Autodesk Fusion 360 part; units mm, degrees
sketch "Sketch1" plane through (0, 0, 0) normal (0, 0, 1) x (1, 0, 0)
  line L0 (-21.8, 22.2397) -> (26.7, 22.2397)
  line L1 (26.7, 22.2397) -> (26.7, -22.7603)
  line L2 (26.7, -22.7603) -> (-21.8, -22.7603)
  line L3 (-21.8, -22.7603) -> (-21.8, 22.2397)
  spline S0 degree 5 poles (-8.2949, 12.4487) (-8.8839, 11.9576) (-10.0102, 10.9741) (-11.5448, 9.495) (-13.2761, 7.5148) (-14.8799, 5.0253) (-15.8741, 2.5205) (-16.2099, -0.001) (-15.8626, -2.5398) (-14.8614, -5.0951) (-13.2565, -7.6657) (-11.5298, -9.7334) (-10.0015, -11.2901) (-8.8808, -12.3304) (-8.2949, -12.8513) knots 0 0 0 0 0 0 0.1 0.2 0.3 0.4 0.5 0.6 0.7 0.8 0.9 1 1 1 1 1 1
  spline S1 degree 5 poles (14.2993, 7.4153) (14.5562, 7.1034) (15.0477, 6.4806) (15.718, 5.5494) (16.4756, 4.3142) (17.1805, 2.7814) (17.6209, 1.2609) (17.7748, -0.2462) (17.6287, -1.7394) (17.193, -3.2192) (16.4888, -4.6864) (15.7281, -5.8511) (15.0535, -6.7197) (14.5583, -7.2967) (14.2993, -7.5847) knots 0 0 0 0 0 0 0.1 0.2 0.3 0.4 0.5 0.6 0.7 0.8 0.9 1 1 1 1 1 1
  line L4 (-21.8, -1.6206) -> (-14.6097, -1.6206)
  line L5 (-14.6097, -1.6206) -> (-14.6097, 0.3794)
  line L6 (-14.6097, 0.3794) -> (-21.8, 0.3794)
  line L7 (14.2993, 7.4153) -> (0.6904, 13.733)
  line L8 (0.6904, 13.733) -> (-8.2949, 12.4487)
  line L9 (0.4715, -12.8513) -> (-8.2949, -12.8513)
  line L10 (14.2993, -7.5847) -> (8.5702, -10.0161)
  line L11 (8.5702, -10.0161) -> (0.4715, -12.8513)
  point P0 (-16.0393, 0.095)
  point P1 (17.6997, -0.3339)
  dimension "d6" = 48.5
  dimension "d7" = 45
  dimension "d8" = 15
  dimension "d9" = 25.3
  dimension "d11" = 2
extrude "Extrude1" add sketch "Sketch1" along normal blind 35.3 contours L0 L1 L2 L3 S0 S1 L4 L6 L7 L8 L9 L10 L11
sketch "bad_sketch" plane through (0, 0, 0) normal (0, 0, 1) x (1, 0, 0)
  line L0 (24.6924, 6.1679) -> (15.4617, 8.9936)
  line L1 (15.4617, 8.9936) -> (5.166, 12.1454)
  line L2 (5.166, 12.1454) -> (-5.166, 12.8182)
  line L3 (-5.166, 12.8182) -> (-14.9618, 9.182)
  line L4 (-14.9618, 9.182) -> (-20.3307, 2.1177)
  line L5 (-20.3307, 2.1177) -> (-20.3307, -2.686)
  line L6 (-20.3307, -2.686) -> (-14.9618, -8.9968)
  line L7 (-14.9618, -8.9968) -> (-10.0639, -11.3515)
  line L8 (-10.0639, -11.3515) -> (-5.166, -12.4818)
  line L9 (-5.166, -12.4818) -> (5.166, -12.4818)
  line L10 (5.166, -12.4818) -> (10.3139, -11.0689)
  line L11 (10.3139, -11.0689) -> (24.6924, -8.2432)
  line L12 (24.6924, -8.2432) -> (28.2717, -1.8383)
  line L13 (28.2717, -1.8383) -> (28.9264, 0.3007)
  line L14 (28.9264, 0.3007) -> (26.482, 5.6201)
  line L15 (26.482, 5.6201) -> (24.6924, 6.1679)
  line L16 (-28.837, -17.65) -> (19.663, -17.65)
  line L17 (19.663, -17.65) -> (19.663, 27.35)
  line L18 (19.663, 27.35) -> (-28.837, 27.35)
  line L19 (-28.837, 27.35) -> (-28.837, -17.65)
  line L20 (-28.837, -1.4888) -> (-19.0112, -1.4888)
  line L21 (-19.0112, -1.4888) -> (-19.0112, 0.5112)
  line L22 (-19.0112, 0.5112) -> (-28.837, 0.5112)
  line L23 (-28.837, 0.5112) -> (-28.837, -1.4888)
  dimension "d15" = 48.5
  dimension "d16" = 45
  dimension "d17" = 2
sketch "Sketch3" plane through (0, 22.2397, 0) normal (0, 1, 0) x (-1, 0, 0)
  line L0 (-26.7, 0) -> (21.8, 0)
  line L1 (21.8, 0) -> (21.8, 35.3)
  line L2 (21.8, 35.3) -> (-26.7, 35.3)
  line L3 (-26.7, 35.3) -> (-26.7, 0)
  circle A0 centre (18.6487, 11.1813) radius 1.7
  line L4 (21.8, 13.5098) -> (16.4, 13.5098)
  line L5 (16.4, 13.5098) -> (16.4, 8.2098)
  line L6 (16.4, 8.2098) -> (21.8, 8.2098)
  line L7 (21.8, 8.2098) -> (21.8, 13.5098)
  dimension "d23" = 3.4
  dimension "d26" = 5.4
  dimension "d27" = 5.3
hole "Hole1" at (-18.6487, 22.2397, 11.1813) direction (0, -1, 0) diameter 3.4 depth 26 tip angle 180
extrude "Extrude3" cut sketch "Sketch3" against normal blind 16 contours L1 L4 L5 L6 L7
sketch "Sketch4" plane through (0, -22.7603, 0) normal (0, -1, 0) x (1, 0, 0)
  line L0 (-21.8, 0) -> (26.7, 0)
  line L1 (26.7, 0) -> (26.7, 35.3)
  line L2 (26.7, 35.3) -> (-21.8, 35.3)
  line L3 (-21.8, 35.3) -> (-21.8, 0)
  line L4 (18.0274, 30.3462) -> (-12.9426, 30.3462)
  line L5 (18.0274, 30.3462) -> (18.0274, 5.3462)
  line L6 (18.0274, 5.3462) -> (-12.9426, 5.3462)
  circle A0 centre (18.0274, 5.3462) radius 1.6
  circle A1 centre (-12.9426, 5.3462) radius 1.6
  circle A2 centre (18.0274, 30.3462) radius 1.6
  circle A3 centre (-12.9426, 30.3462) radius 1.6
  line L7 (26.7, 14.5722) -> (17.935, 14.5722)
  dimension "d36" = 30.97
  dimension "d38" = 25
  dimension "d40" = 30.97
  dimension "d41" = 3.2
  dimension "d42" = 3.2
  dimension "d43" = 3.2
  dimension "d44" = 3.2
  dimension "d45" = 8.765
hole "Hole2" at (18.0274, -22.7603, 5.3462) at (-12.9426, -22.7603, 5.3462) at (18.0274, -22.7603, 30.3462) at (-12.9426, -22.7603, 30.3462) direction (0, 1, 0) diameter 3.2 depth 12 tip angle 180
sketch "Sketch5" plane through (-21.8, 0, 0) normal (-1, 0, 0) x (0, -1, 0)
  line L0 (1.6206, 0) -> (22.7603, 0)
  line L1 (22.7603, 0) -> (22.7603, 35.3)
  line L2 (22.7603, 35.3) -> (1.6206, 35.3)
  line L3 (1.6206, 35.3) -> (1.6206, 0)
  line L4 (22.7603, 16.2062) -> (19.7603, 16.2062)
  line L5 (19.7603, 7.0647) -> (16.0603, 7.0647)
  line L6 (16.0603, 7.0647) -> (16.0603, 1.8647)
  line L7 (16.0603, 1.8647) -> (19.7603, 1.8647)
  line L8 (19.7603, 1.8647) -> (19.7603, 7.0647)
  line L9 (19.7603, 27.5787) -> (16.0603, 27.5787)
  line L10 (16.0603, 27.5787) -> (16.0603, 32.7787)
  line L11 (16.0603, 32.7787) -> (19.7603, 32.7787)
  line L12 (19.7603, 32.7787) -> (19.7603, 27.5787)
  line L13 (6.4749, 8.7948) -> (2.7749, 8.7948)
  line L14 (2.7749, 8.7948) -> (2.7749, 13.9948)
  line L15 (2.7749, 13.9948) -> (6.4749, 13.9948)
  line L16 (6.4749, 13.9948) -> (6.4749, 8.7948)
  dimension "d55" = 3
  dimension "d56" = 3.7
  dimension "d57" = 5.2
  dimension "d58" = 3.7
  dimension "d59" = 5.2
  dimension "d65" = 3.7
  dimension "d66" = 5.2
extrude "Extrude4" cut sketch "Sketch5" against normal blind 12 contours L9 L10 L11 L12
extrude "Extrude5" cut sketch "Sketch5" against normal blind 12 contours L5 L6 L7 L8
extrude "Extrude6" cut sketch "Sketch5" against normal blind 5.4 contours L13 L14 L15 L16
sketch "Sketch7" plane through (26.7, 0, 0) normal (1, 0, 0) x (0, 1, 0)
  line L0 (-22.7603, 0) -> (22.2397, 0)
  line L1 (22.2397, 0) -> (22.2397, 35.3)
  line L2 (22.2397, 35.3) -> (-22.7603, 35.3)
  line L3 (-22.7603, 35.3) -> (-22.7603, 0)
  line L4 (-19.7634, 32.4808) -> (-16.0634, 32.4808)
  line L5 (-16.0634, 32.4808) -> (-16.0634, 27.2808)
  line L6 (-16.0634, 27.2808) -> (-19.7634, 27.2808)
  line L7 (-19.7634, 27.2808) -> (-19.7634, 32.4808)
  line L8 (-19.7359, 7.0548) -> (-16.0359, 7.0548)
  line L9 (-16.0359, 7.0548) -> (-16.0359, 1.8548)
  line L10 (-16.0359, 1.8548) -> (-19.7359, 1.8548)
  line L11 (-19.7359, 1.8548) -> (-19.7359, 7.0548)
  dimension "d76" = 3.7
  dimension "d77" = 5.2
  dimension "d78" = 3.7
  dimension "d79" = 5.2
extrude "Extrude8" cut sketch "Sketch7" against normal blind 12 contours L4 L5 L6 L7 | L8 L9 L10 L11
equation "syringe_height = 25.3 mm"
equation "syringe_width = 33.6 mm"
equation "height = 45 mm"
equation "width = 48.5 mm"
equation "width4 = 15 mm"
equation "d6 = width"
equation "d7 = height"
equation "d8 = width4"
equation "d9 = syringe_height"
equation "gap_width = 2 mm"
equation "d11 = gap_width"
equation "d12 = holder_depth"
equation "d15 = width"
equation "d16 = height"
equation "d17 = gap_width"
equation "length = 3 mm"
equation "holder_depth = 35.3 mm"
equation "m3_screw_diameter = 3.4 mm"
equation "d23 = m3_screw_diameter"
equation "rect_clearing_width = 5.3 mm"
equation "rect_clearing_length = 5.4 mm"
equation "d26 = rect_clearing_length"
equation "d27 = rect_clearing_width"
equation "d28 = joining_m3_screw_length"
equation "d29 = m3_screw_diameter"
equation "joining_m3_screw_length = 26 mm"
equation "rect_clearing_distance = 16 mm"
equation "m3_screw_lateral_dis = 30.97 mm"
equation "d36 = m3_screw_lateral_dis"
equation "m3_screw_vertical_dis = 25 mm"
equation "d38 = m3_screw_vertical_dis"
equation "m3_diameter = 3.2 mm"
equation "d40 = m3_screw_lateral_dis"
equation "d41 = m3_diameter"
equation "d42 = m3_diameter"
equation "d43 = m3_diameter"
equation "d44 = m3_diameter"
equation "d46 = m3_screw_depth"
equation "d47 = m3_diameter"
equation "m3_screw_depth = 12 mm"
equation "nut_insert_width = 3.7 mm"
equation "nut_insert_height = 5.2 mm"
equation "screw_nut_distance = 3 mm"
equation "d55 = screw_nut_distance"
equation "d56 = nut_insert_width"
equation "d57 = nut_insert_height"
equation "d58 = nut_insert_width"
equation "d59 = nut_insert_height"
equation "d60 = -m3_screw_depth"
equation "d62 = -m3_screw_depth"
equation "d65 = nut_insert_width"
equation "d66 = nut_insert_height"
equation "clamp_nut_depth = 5.4 mm"
equation "d76 = nut_insert_width"
equation "d77 = nut_insert_height"
equation "d78 = nut_insert_width"
equation "d79 = nut_insert_height"
equation "d80 = -m3_screw_depth"
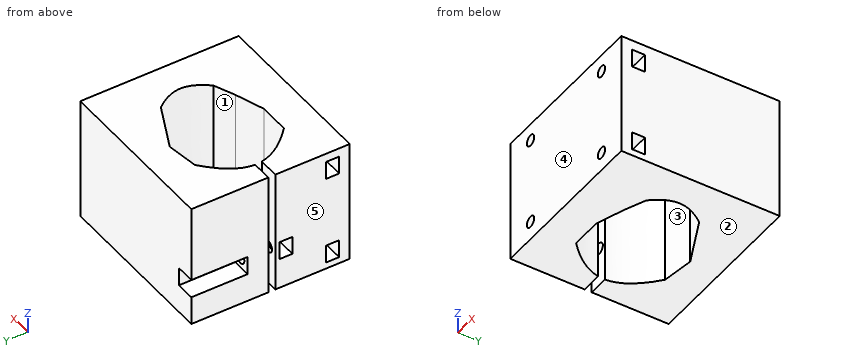
Verification items for the finished model (mm, model axes). Face numbers are marked on the shaded views. A direction names the side the tool comes from. Coordinates: 2 decimals unless noted, no trailing zeros. Order: outer loops, then holes, each group sorted by start corner. A loop starts at its lowest first (then second) coordinate and runs counter-clockwise, first axis right, second up. Notation, with made-up numbers: M 5.25,-21 L 64.25,-21 A19 ccw 64.25,6 Z; hole C 88.5,-9 d10. An arc over 180 degrees is marked long. One line per item, written item: value. Start each with the question number.
Item 1: Mould release check, pull along X, two halves, no side actions. Record for the marked faces 3, 4 and 5: released by +X, released by -X, zero draft, split by the parting line, or undercut.
Item 2: Access from +Z, -Z, +X, -X, +Y, -Y to the whole of each face (thin tool, end or side, straight path). Record for the marked faces 1 and 2.
Item 3: Scan lines: probe 1 along X at (y, z) = (-20, 31); probe 2 along Y at (x, z) = (-8, 9); probe 3 along Y at (x, z) = (10, 19). Record each from-to range of solid material in increasing order.
Item 4: Sectioned sample at A-A (x = 23). Enter the section's corners in (y, z), then the cut area to 3 significant figures.
Item 5: Sectioned sample at B-B (y = 15). Enter the section's corners in (x, z).
Item 6: Sectioned sample at C-C (x = 6.5). Enter the section's corners in (y, z).
Item 7: Sectioned sample at D-D (y = -15). Enter the section's corners in (x, z), then the cut area to 3 significant figures.
Item 8: Gauge pin test, flat ends, axial feed: pin 1 (6 mm diameter, centred on x = -12.5, y = 7.5, fed in from -Z); pin 2 (3 mm diameter, centred on y = -18, z = 30, fed in from -X). Record the tip position at first contact, or that the pin passes through.
Conclusion:
1. face 3: undercut
1. face 4: zero draft
1. face 5: released by -X
2. face 1: +Z, -Z
2. face 2: -Z, +X, -X, +Y, -Y
3. probe 1: x = -21.8 to -14.4, -11.48 to 16.57, 19.49 to 26.7
3. probe 2: y = -22.76 to -12.85, 12.49 to 22.24
3. probe 3: y = -22.76 to -9.41, 9.41 to 22.24
4. outline: M -22.76,0 L 22.24,0 L 22.24,35.3 L -22.76,35.3 Z; hole M -19.76,27.28 L -16.06,27.28 L -16.06,32.48 L -19.76,32.48 Z; hole M -19.74,1.85 L -16.04,1.85 L -16.04,7.05 L -19.74,7.05 Z
4. area: 1,550 mm^2
5. outline: M -21.8,0 L 26.7,0 L 26.7,35.3 L -21.8,35.3 L -21.8,13.51 L -16.4,13.51 L -16.4,8.21 L -21.8,8.21 Z
6. outline: M -22.76,0 L -10.74,0 L -10.74,35.3 L -22.76,35.3 Z; M 11.04,0 L 22.24,0 L 22.24,35.3 L 11.04,35.3 Z
7. outline: M -21.8,0 L 26.7,0 L 26.7,35.3 L -21.8,35.3 Z; hole C -12.94,5.35 d3.2; hole C -12.94,30.35 d3.2; hole C 18.03,5.35 d3.2; hole C 18.03,30.35 d3.2
7. area: 1,680 mm^2
8. pin 1: stops at z = 0
8. pin 2: stops at x = -9.8
